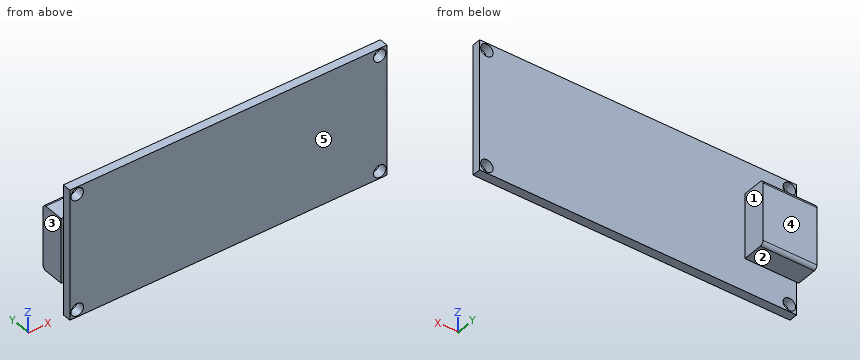
```python
from build123d import *

# Parameters (mm, degrees)
SKETCH1_W           = 43.5
SKETCH1_H           = 17.9
SKETCH1_R           = 0.85
BOSS_EXTRUDE1_DEPTH = 1.2
SKETCH2_W           = 7.4
SKETCH2_H           = 8.9
BOSS_EXTRUDE2_DEPTH = 3.3
FILLET1_R           = 0.5


with BuildPart() as part:
    # Sketch1 → Boss-Extrude1 (new body)
    with BuildSketch(Plane(origin=(0, 0, 0), x_dir=(1, 0, 0), z_dir=(0, 1, 0))):
        Rectangle(SKETCH1_W, SKETCH1_H)
        with Locations(Location((-20.75, 7.95, 0), (0, 0, 270))):
            Circle(SKETCH1_R, mode=Mode.SUBTRACT)
        with Locations(Location((20.75, -7.95, 0), (0, 0, 270))):
            Circle(SKETCH1_R, mode=Mode.SUBTRACT)
        with Locations(Location((20.75, 7.95, 0), (0, 0, 270))):
            Circle(SKETCH1_R, mode=Mode.SUBTRACT)
        with Locations(Location((-20.75, -7.95, 0), (0, 0, 270))):
            Circle(SKETCH1_R, mode=Mode.SUBTRACT)
    extrude(amount=BOSS_EXTRUDE1_DEPTH)

    # Sketch2 → Boss-Extrude2 (add)
    with BuildSketch(Plane(origin=(0, 1.2, 0), x_dir=(1, 0, 0), z_dir=(0, 1, 0))):
        with Locations((-18.35, 0)):
            Rectangle(SKETCH2_W, SKETCH2_H)
    extrude(amount=BOSS_EXTRUDE2_DEPTH)

    # Fillet1
    fillet1_edges = [part.edges().sort_by_distance(p)[0] for p in [
        (-18.35, 4.5, 4.45),
        (-18.35, 4.5, -4.45),
    ]]
    fillet(fillet1_edges, radius=FILLET1_R)


solid = part.part
```
The listing builds one solid part. Answer for the finished solid, in the listing's coordinates (mm). Face numbers are marked on the shaded views. A direction names the side the tool comes from. Give positions to 0.01 mm unless a question says otherwise; leave off trailing zeros. Order: outer loops, then holes, each group sorted by start corner. A loop starts at its lowest first (then second) coordinate and runs counter-clockwise, first axis right, second up. Notation, with made-up numbers: (-21, 39) -> (20, 39) arc R10 ccw to (20, 44) -> close; hole circle Ø1 at (-26, 60). An arc over 180 degrees is marked (long way). Answer as a JSON object with one key per item and string values. Group by question number.
Item 1: The part is cut by section B-B on x = 20.75. Write down the section's boundary in (y, z).
Item 2: The part is cut by section A-A on z = 7.95. Write down the section's boundary in (x, y).
Item 3: Flat-ended cylindrical pins translate along their axes: pin 1 (8 mm diameter, centred on x = 14, z = 0.5, fed in from +Y); pin 2 (1.5 mm diameter, centred on x = 20.75, z = -7.95, fed in from -Y); pin 3 (0.8 mm diameter, centred on x = -17, y = 3, fed in from +Z); pin 4 (1 mm diameter, centred on y = 0.5, z = -1, fed in from -X). Find the tip coordinate at first contact, or state that the pin passes through.
Item 4: Consider L1, parallel to X at y = 0.75, z = -7.95; L2, parallel to Z at x = 20.5, y = 0.8; L3, parallel to Y at x = 4.5, z = -3.5. Determine where each line is inside the solid, lowest interval first. Write a range as from..to.
Item 5: The part is cut by section C-C on y = 0.6. Write down the section's boundary in (x, z).
Item 6: A tool of negligible diameter and unlimited length cuts with its end or side. For the marked faces 1 and 2, from which of +Z, -Z, +X, -X, +Y, -Y can it reach the whole face along a straight path? Write none if from no direction.
Item 7: The part is cut by section D-D on z = -1.5. Write down the section's boundary in (x, y), and give its area (3 significant figures).
Item 8: Determine the mould class of the marked faces 3, 4 and 5 for opening direction Y: pulls with the +Y half, pulls with the -Y half, needs draft (parallel to the pull), parting line crosses it, or undercut.
Result set:
{
 "1": {"outline": "(0, -8.95) -> (1.2, -8.95) -> (1.2, -8.8) -> (0, -8.8) -> close; (0, -7.1) -> (1.2, -7.1) -> (1.2, 7.1) -> (0, 7.1) -> close; (0, 8.8) -> (1.2, 8.8) -> (1.2, 8.95) -> (0, 8.95) -> close"},
 "2": {"outline": "(-21.75, 0) -> (-21.6, 0) -> (-21.6, 1.2) -> (-21.75, 1.2) -> close; (-19.9, 0) -> (19.9, 0) -> (19.9, 1.2) -> (-19.9, 1.2) -> close; (21.6, 0) -> (21.75, 0) -> (21.75, 1.2) -> (21.6, 1.2) -> close"},
 "3": {"pin 1": "y = 1.2", "pin 2": "through", "pin 3": "z = 4.45", "pin 4": "x = -21.75"},
 "4": {"L1": "-21.75..-21.6, -19.9..19.9, 21.6..21.75", "L2": "-8.95..-8.76, -7.14..7.14, 8.76..8.95", "L3": "0..1.2"},
 "5": {"outline": "(-21.75, -8.95) -> (21.75, -8.95) -> (21.75, 8.95) -> (-21.75, 8.95) -> close; hole circle Ø1.7 at (-20.75, -7.95); hole circle Ø1.7 at (-20.75, 7.95); hole circle Ø1.7 at (20.75, -7.95); hole circle Ø1.7 at (20.75, 7.95)"},
 "6": {"face 1": "+Z, -Z, +X, +Y", "face 2": "-Z, +X, -X, +Y"},
 "7": {"outline": "(-22.05, 1.2) -> (-21.75, 1.2) -> (-21.75, 0) -> (21.75, 0) -> (21.75, 1.2) -> (-14.65, 1.2) -> (-14.65, 4.5) -> (-22.05, 4.5) -> close", "area": "76.6 mm²"},
 "8": {"face 3": "needs draft", "face 4": "pulls with the +Y half", "face 5": "pulls with the -Y half"}
}
